Geometry check sheet. Reference: the model listing, model coordinates, mm. A direction names the side the tool comes from. Give positions to 0.01 mm unless a question says otherwise; leave off trailing zeros. Write each loop counter-clockwise with the first axis right and the second up, starting at its lowest first coordinate (ties: lowest second). Pieces come first, ordered by that corner, then holes. Notation, with made-up numbers: M 74.5,55 L 110.5,55 A24 cw 110.5,79 Z; hole C 0.5,46.25 d10. An arc over 180 degrees is marked long. Write each question's results on one line, items separated by ' | '.
```python
from build123d import *

# Parameters (mm, degrees)
SKETCH1_W           = 60.198
SKETCH1_H           = 85.725
SKETCH1_R           = 3.175
BOSS_EXTRUDE1_DEPTH = 12.7
SKETCH3_R           = 4.7625
BOSS_EXTRUDE2_DEPTH = 7.9375
BOSS_EXTRUDE3_DEPTH = 3.175
BOSS_EXTRUDE4_DEPTH = 3.175
FILLET1_R           = 2.54
CHAMFER1_SIZE       = 2.54
SKETCH15_R          = 2.54
CUT_EXTRUDE1_DEPTH  = 12.7


with BuildPart() as part:
    # Sketch1 → Boss-Extrude1 (new body)
    with BuildSketch(Plane(origin=(0, 0, 0), x_dir=(0, 0, -1), z_dir=(1, 0, 0))):
        with Locations((30.099, 42.8625)):
            Rectangle(SKETCH1_W, SKETCH1_H)
        with Locations((50.673, 58.7375)):
            Circle(SKETCH1_R, mode=Mode.SUBTRACT)
    extrude(amount=-BOSS_EXTRUDE1_DEPTH)

    # Sketch3 → Boss-Extrude2 (add)
    with BuildSketch(Plane(origin=(0, 0, 0), x_dir=(0, 0, -1), z_dir=(1, 0, 0))):
        with Locations((25.4, 57.15)):
            Circle(SKETCH3_R)
        Polygon((18.923, 39.573522628), (25.273, 28.575), (14.274477372, 22.225), (7.924477372, 33.223522628), align=None)
        with BuildLine():
            Line((56.355023328, 81.24857189), (46.259909872, 65.09335031))
            ThreePointArc((46.259909872, 65.09335031), (43.22985581, 78.218517828), (56.355023328, 81.24857189))
        make_face()
    extrude(amount=BOSS_EXTRUDE2_DEPTH)

    # Sketch10 → Boss-Extrude3 (add)
    with BuildSketch(Plane(origin=(7.9375, 0, 0), x_dir=(0, 0, -1), z_dir=(1, 0, 0))):
        Polygon((26.305931595, 66.631820128), (17.641468693, 62.67546984), (16.735537097, 53.193649712), (24.494068405, 47.668179872), (33.158531307, 51.62453016), (34.064462903, 61.106350288), align=None)
    extrude(amount=BOSS_EXTRUDE3_DEPTH)

    # Sketch14 → Boss-Extrude4 (add)
    with BuildSketch(Plane(origin=(7.9375, 0, 0), x_dir=(0, 0, -1), z_dir=(1, 0, 0))):
        Polygon((51.3074666, 73.1709611), (58.881956407, 85.29242578), (46.18969706, 85.735768391), (37.770793083, 72.262986752), (43.732976793, 61.04949642), align=None)
    extrude(amount=BOSS_EXTRUDE4_DEPTH)

    # Fillet1
    fillet1_edges = [part.edges().sort_by_distance(p)[0] for p in [
        (3.96875, 39.573522628, -18.923),
        (3.96875, 33.223522628, -7.924477372),
        (3.96875, 22.225, -14.274477372),
        (3.96875, 28.575, -25.273),
        (9.525, 61.106350288, -34.064462903),
        (9.525, 66.631820128, -26.305931595),
        (9.525, 62.67546984, -17.641468693),
        (9.525, 53.193649712, -16.735537097),
        (9.525, 47.668179872, -24.494068405),
        (9.525, 51.62453016, -33.158531307),
        (9.525, 61.04949642, -43.732976793),
        (9.525, 85.29242578, -58.881956407),
        (9.525, 85.735768391, -46.18969706),
        (9.525, 72.262986752, -37.770793083),
    ]]
    fillet(fillet1_edges, radius=FILLET1_R)

    # Chamfer1
    chamfer1_edges = [part.edges().sort_by_distance(p)[0] for p in [
        (0, 57.15, -20.6375),
        (0, 78.218517828, -43.22985581),
    ]]
    chamfer(chamfer1_edges, length=CHAMFER1_SIZE)

    # Sketch15 → Cut-Extrude1 (cut)
    with BuildSketch(Plane(origin=(0, 18.087280015, -31.328087957), x_dir=(-1, 0, 0), z_dir=(0, 0.5, -0.866025404))):
        with Locations((-4.114917268, 18.460175913)):
            Circle(SKETCH15_R)
    extrude(amount=-CUT_EXTRUDE1_DEPTH, mode=Mode.SUBTRACT)


solid = part.part
```
Q1. Depth check by flat-ended pin: P1, Ø10, axis at y = 58.74, z = -50.67, coming from the +X side; P2, Ø1, axis at x = 2, y = 38, coming from the +Z side; P3, Ø7.5, axis at y = 31.5, z = -20, coming from the +X side. Enter the tip coordinate at first touch or a pass-through.
Answer key:
P1: stops at x = 0 | P2: stops at z = -15.33 | P3: stops at x = 7.94
Q2. Material ranges on probe 1 along X at (y, z) = (77.5, -24); probe 2 along Z at (x, y) = (-4, 56.5); probe 3 along Y at (x, z) = (2.25, -15), recorded low to high. Write a range as [from, to].
Answer key:
probe 1: x = [-12.7, 0] | probe 2: z = [-60.2, -52.93], [-48.42, 0] | probe 3: y = [23.16, 27.99], [31.97, 37.31]
Q3. Release check for a two-part mould opening along Z. For faces 1 (the face through (9.5, 62.5, -18)), 2 (the face through (-6, 42, -60.198)), 3 (the face through (9.547, 66.242, -26.25)), 4 (the face through (9.547, 63.587, -43.859)) record: released by +Z, released by -Z, zero draft, split by the parting line, or undercut.
Answer key:
face 1: released by +Z | face 2: released by -Z | face 3: undercut | face 4: undercut
Q4. Access from +Z, -Z, +X, -X, +Y, -Y to the whole of each face (thin tool, end or side, straight path). Record for faces 5 (the face through (7.938, 31, -17)), 6 (the face through (4.02, 32.98, -8.95)), 7 (the face through (2.38, 78.12, -42.98)), 8 (the face through (9.55, 51.87, -32.85)), 9 (the face through (1.27, 34.12, -22.07)).
Answer key:
face 5: +Z, -Z, +X, -Y | face 6: +Z, +X | face 7: none | face 8: -Z, +X, -Y | face 9: -Z, +X
Q5. Section check B-B (x = 4.25). State how many separate pieces and enclosed holes the cut face has, then the cut area to 3 significant figures.
Answer key:
separate pieces: 4 | enclosed holes: 0 | area: 305 mm2
Q6. Section check A-A (y = 57.15). Enter the section's corners in (x, z), then the cut area to 3 significant figures.
Answer key:
outline: M -12.7,-60.2 L 0,-60.2 L 0,-53.42 L -12.7,-53.42 Z; M -12.7,-47.92 L 0,-47.92 L 0,-32.7 L 2.54,-30.16 L 7.94,-30.16 L 7.94,-33.69 L 11.11,-33.69 L 11.11,-17.11 L 7.94,-17.11 L 7.94,-20.64 L 2.54,-20.64 L 0,-18.1 L 0,0 L -12.7,0 Z | area: 829 mm2
